from build123d import *

# Parameters (mm, degrees)
BOSS_EXTRUDE1_DEPTH = 2.5


with BuildPart() as part:
    # Sketch1 → Boss-Extrude1 (new body)
    with BuildSketch(Plane(origin=(0, 0, 0), x_dir=(0, 0, -1), z_dir=(1, 0, 0))):
        Polygon((100, 20), (20, 110), (0, 110), (0, 102.2), (5, 102.2), (5, 103.85), (9, 103.85), (9, 102.2), (11.5, 102.2), (11.5, 97.8), (9, 97.8), (9, 96.15), (5, 96.15), (5, 97.8), (0, 97.8), (0, 85), (-5, 85), (-5, 75), (0, 75), (0, 32.2), (5, 32.2), (5, 33.85), (9, 33.85), (9, 32.2), (11.5, 32.2), (11.5, 27.8), (9, 27.8), (9, 26.15), (5, 26.15), (5, 27.8), (0, 27.8), (0, 20), (-5, 20), (-5, 0), (0, 0), (0, -5), (20, -5), (20, 0), (82.8, 0), (82.8, 5), (81.15, 5), (81.15, 9), (82.8, 9), (82.8, 11.5), (87.2, 11.5), (87.2, 9), (88.85, 9), (88.85, 5), (87.2, 5), (87.2, 0), (100, 0), align=None)
    extrude(amount=BOSS_EXTRUDE1_DEPTH)


solid = part.part
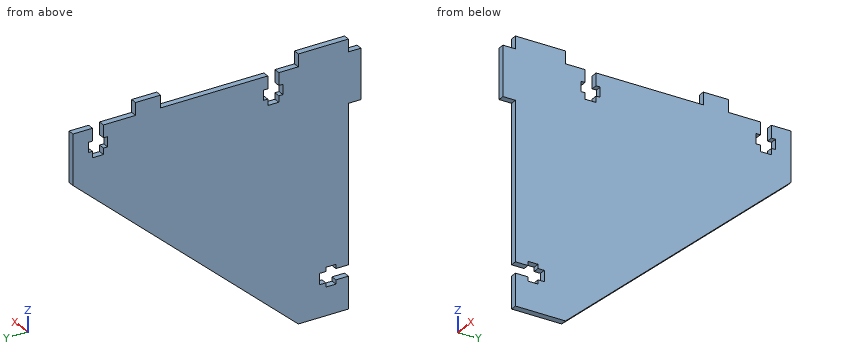
Here's how the part is built. I have some questions about the finished solid (model axes, mm). Round coordinates to 2 decimals unless told otherwise and drop trailing zeros. Order: outer loops, then holes, each group sorted by start corner. A loop starts at its lowest first (then second) coordinate and runs counter-clockwise, first axis right, second up. Notation, with made-up numbers: M -5.75,-14.75 L 36.25,-14.75 A19 cw 36.25,12.25 Z; hole C 49,39.5 d10. An arc over 180 degrees is marked long. One line per question, with ' | ' between items.
1) I'm going to push flat-ended pins straight in: pin 1 Ø0.8 at (x, z) = (1, -88) entering from -Y; pin 2 Ø0.5 at (x, y) = (1.5, 97) entering from -Z; pin 3 Ø1.2 at (x, y) = (1, -2.5) entering from +Z. Where does each tip first touch, or does it pass through?
Checked values:
pin 1: stops at y = 0 | pin 2: stops at z = -31.78 | pin 3: stops at z = 0
2) I need wall thicknesses on line 1 (Y direction, x = 2.1, z = -10); line 2 (Z direction, x = 2.45, y = 33); line 3 (Y direction, x = 1.2, z = -57) (3 decimals). Which ranges of each line are inside material? Lowest first, please.
Checked values:
line 1: y = -5 to 27.8, 32.2 to 97.8, 102.2 to 110 | line 2: z = -88.44 to -9, -5 to 0 | line 3: y = 0 to 68.375
3) Imagine slicing it at B-B, the plane z = -40. Write out the boundary of the cut face in (x, y), plus the area to 3 significant figures.
Checked values:
outline: M 0,0 L 2.5,0 L 2.5,87.5 L 0,87.5 Z | area: 219 mm²
4) Imagine slicing it at A-A, the plane z = -3. Write out the boundary of the cut face in (x, y).
Checked values:
outline: M 0,-5 L 2.5,-5 L 2.5,27.8 L 0,27.8 Z; M 0,32.2 L 2.5,32.2 L 2.5,97.8 L 0,97.8 Z; M 0,102.2 L 2.5,102.2 L 2.5,110 L 0,110 Z
5) Imagine slicing it at C-C, the plane y = 60. Write out the boundary of the cut face in (x, z), plus the area to 3 significant figures.
Checked values:
outline: M 0,-64.44 L 2.5,-64.44 L 2.5,0 L 0,0 Z | area: 161 mm²
